Build history of the part. All positions in model axes, mm. A direction names the side the tool comes from. Round coordinates to 2 decimals unless told otherwise and drop trailing zeros. Order: outer loops, then holes, each group sorted by start corner. A loop starts at its lowest first (then second) coordinate and runs counter-clockwise, first axis right, second up. Notation, with made-up numbers: (50, -28) -> (93, -28) arc R15 ccw to (93, -1) -> close; hole circle Ø2 at (12, 57.5). An arc over 180 degrees is marked (long way). Answer as a JSON object with one key per item and string values.
Autodesk Inventor part; units mm, degrees
ref_plane "nut_to_bolt_XY" through (0, 0, 3) normal (0, 1, 0) x (1, 0, 0)
ref_plane "nut_to_bolt_YZ" through (0, 0, 3) normal (1, 0, 0) x (0, 0, -1)
ref_plane "nut_to_bolt_ZX" through (0, 0, 3) normal (0, 0, -1) x (0, 1, 0)
sketch "Sketch_1" plane through (0, 0, 0) normal (0, 0, 1) x (1, 0, 0)
  arc A0 (-3.35, 0) -> (-3.7968, -0.7244) centre (-3.35, -0.5) ccw
  line L0 (-3.7968, -0.7244) -> (-3.5468, -1.2222)
  arc A1 (-3.5468, -1.2222) -> (-1.1318, -4.0103) centre (3.1555, 2.1435) ccw
  arc A2 (-1.1318, -4.0103) -> (-0.846, -4.1) centre (-0.846, -3.6) ccw
  line L1 (-0.846, -4.1) -> (0.846, -4.1)
  arc A3 (0.846, -4.1) -> (1.1318, -4.0103) centre (0.846, -3.6) ccw
  arc A4 (1.1318, -4.0103) -> (3.5468, -1.2222) centre (-3.1555, 2.1435) ccw
  line L2 (3.5468, -1.2222) -> (3.7968, -0.7244)
  arc A5 (3.7968, -0.7244) -> (3.35, 0) centre (3.35, -0.5) ccw
  line L3 (3.35, 0) -> (2.7, 0)
  arc A6 (2.5, 0.2) -> (2.7, 0) centre (2.7, 0.2) ccw
  line L4 (2.5, 0.2) -> (2.5, 0.4)
  arc A7 (2.5, 0.4) -> (2.3, 0.6) centre (2.3, 0.4) ccw
  line L5 (2.3, 0.6) -> (-2.3, 0.6)
  arc A8 (-2.3, 0.6) -> (-2.5, 0.4) centre (-2.3, 0.4) ccw
  line L6 (-2.5, 0.4) -> (-2.5, 0.2)
  arc A9 (-2.7, 0) -> (-2.5, 0.2) centre (-2.7, 0.2) ccw
  line L7 (-2.7, 0) -> (-3.35, 0)
extrude "Extrusion1" add sketch "Sketch_1" along normal mid plane 12
sketch "Sketch_2" plane through (0, 0, 0) normal (1, 0, 0) x (0, 1, 0)
  line L0 (0.6, 3) -> (-4.1, 3)
  line L1 (-4.1, 3) -> (-4.1, 5.5)
  line L2 (-4.1, 5.5) -> (-3.667, 5.067)
  line L3 (-3.667, 5.067) -> (0.167, 5.067)
  line L4 (0.167, 5.067) -> (0.6, 5.5)
  line L5 (0.6, 5.5) -> (0.6, 3)
  line L6 (0.6, 3) -> (-4.1, 3)
revolve "Revolution1" cut sketch "Sketch_2" angle 360 about axis through (0, 0.6, 3) along (0, 1, 0)
thread "Thread1"
sketch "Sketch3" plane through (-0.846, -4.1, -6) normal (0, -1, 0) x (1, 0, 0)
  point P0 (0.846, 3)
hole "Hole1" at (0, -4.1, -3) direction (0, 1, 0) diameter 3 depth 3.28
sketch "Sketch_5" plane through (0, 0, 0) normal (1, 0, 0) x (0, 1, 0)
  line L0 (-3.449, -1.499) -> (-3.449, -4.501)
  arc A0 (-3.449, -1.499) -> (-3.449, -4.501) centre (-3.449, -3) ccw
  line L1 (-3.449, -1.499) -> (-3.449, -4.501)
revolve "Revolution2" add sketch "Sketch_5" angle 360 about axis through (0, -3.449, -1.499) along (0, 0, 1)
ref_plane "nut_to_bolt_XY" through (0, 0, 3) normal (0, 1, 0) x (1, 0, 0)
ref_plane "nut_to_bolt_YZ" through (0, 0, 3) normal (1, 0, 0) x (0, 0, -1)
ref_plane "nut_to_bolt_ZX" through (0, 0, 3) normal (0, 0, -1) x (0, 1, 0)
properties part number "13084_m"
1) Cut at D-D, the plane z = -0.25. Give the cut face in (x, y).
Checked values:
{"outline": "(-3.8, -0.72) -> (-3.55, -1.22) arc R7.5 ccw to (-1.13, -4.01) arc R0.5 ccw to (-0.85, -4.1) -> (0.85, -4.1) arc R0.5 ccw to (1.13, -4.01) arc R7.5 ccw to (3.55, -1.22) -> (3.8, -0.72) arc R0.5 ccw to (3.35, 0) -> (2.7, 0) arc R0.2 cw to (2.5, 0.2) -> (2.5, 0.4) arc R0.2 ccw to (2.3, 0.6) -> (-2.3, 0.6) arc R0.2 ccw to (-2.5, 0.4) -> (-2.5, 0.2) arc R0.2 cw to (-2.7, 0) -> (-3.35, 0) arc R0.5 ccw to start"}
2) Probe L1, parallel to Z at x = 0.75, y = -1.5; L2, parallel to Z at x = 0, y = -2.7; L3, parallel to X at y = -2, z = 3. List the from-to ranges inside material, lowest first. Write a range as from..to.
Checked values:
{"L1": "z = -6..-4.3, -1.7..1.07, 4.93..6", "L2": "z = -6..-4.5, -4.3..-1.7, -1.5..0.93, 5.07..6", "L3": "x = -3.1..-2.07, 2.07..3.1"}
3) Cut at C-C, the plane y = -2.9. Give the cut face in (x, z), plus the area to 3 significant figures.
Checked values:
{"outline": "(-2.4, -6) -> (2.4, -6) -> (2.4, 6) -> (-2.4, 6) -> close; circle Ø2.79 at (0, -3); hole circle Ø4.13 at (0, 3); hole circle Ø3 at (0, -3)", "area": "43.1 mm²"}
4) Cut at A-A, the plane x = 0. Give the cut face in (y, z), plus the area to 3 significant figures.
Checked values:
{"outline": "(-4.1, -6) -> (0.6, -6) -> (0.6, 0.5) -> (0.17, 0.93) -> (-3.67, 0.93) -> (-4.1, 0.5) -> (-4.1, -1.5) -> (-3.5, -1.5) arc R1.5 ccw to (-3.5, -4.5) -> (-4.1, -4.5) -> close; (-4.1, 5.5) -> (-3.67, 5.07) -> (0.17, 5.07) -> (0.6, 5.5) -> (0.6, 6) -> (-4.1, 6) -> close; hole (-3.39, -4.5) -> (-0.82, -4.5) -> (-0.82, -1.5) -> (-3.39, -1.5) arc R1.5 cw to start", "area": "33.8 mm²"}
5) Cut at B-B, the plane z = 3. Give the cut face in (x, y).
Checked values:
{"outline": "(-3.8, -0.72) -> (-3.55, -1.22) arc R7.5 ccw to (-2.07, -3.24) -> (-2.07, 0.17) -> (-2.44, 0.54) arc R0.2 ccw to (-2.5, 0.4) -> (-2.5, 0.2) arc R0.2 cw to (-2.7, 0) -> (-3.35, 0) arc R0.5 ccw to start; (2.07, -3.24) arc R7.5 ccw to (3.55, -1.22) -> (3.8, -0.72) arc R0.5 ccw to (3.35, 0) -> (2.7, 0) arc R0.2 cw to (2.5, 0.2) -> (2.5, 0.4) arc R0.2 ccw to (2.44, 0.54) -> (2.07, 0.17) -> close"}
6) Pull direction X, two halves, no side cores. Call faces 1 (the face through (0, -0.82, -3)), 2 (the face through (0, -2, -6)), 3 (the face through (0, -3.8, 0.8)), 4 (the face through (-2.496, -2.787, -0.084)): pulls with the +X half, pulls with the -X half, needs draft (parallel to the pull), parting line crosses it, or undercut.
Checked values:
{"face 1": "undercut", "face 2": "needs draft", "face 3": "undercut", "face 4": "pulls with the -X half"}
7) Flat gauge pins, fed straight in: pin 1 Ø1.9 at (x, z) = (0, 0) entering from -Y; pin 2 Ø0.5 at (x, z) = (-3, 0.5) entering from +Y; pin 3 Ø4 at (x, z) = (2, 2) entering from +Y; pin 4 Ø1 at (y, z) = (-1.5, 3) entering from -X. Where does each tip first touch, or does it go through?
Checked values:
{"pin 1": "stops at y = -4.1", "pin 2": "stops at y = 0", "pin 3": "stops at y = 0.6", "pin 4": "stops at x = -3.66"}
8) Which spindle directions (+Z, -Z, +X, -X, +Y, -Y) get a long thin tool onto all of the face, cutting with end or side? Do faces 5 (the face through (0, -3.8, 5.2)), 6 (the face through (0.03, 0.6, 5.65)), 7 (the face through (0.575, -2.089, -4.386)). Say none if no direction does.
Checked values:
{"face 5": "-Y", "face 6": "+Z, -Z, +X, -X, +Y", "face 7": "none"}
